Can you work these out from the model? Positions are in its coordinate system, mm. A direction names the side the tool comes from. Give positions to 0.01 mm unless a question says otherwise; leave off trailing zeros. Return JSON: item names as keys, results as strings.
```python
from build123d import *

# Parameters (mm, degrees)
SKETCH1_R           = 1.5
SKETCH1_W           = 8
SKETCH1_H           = 8
BOSS_EXTRUDE1_DEPTH = 8.4


with BuildPart() as part:
    # Sketch1 → Boss-Extrude1 (new body)
    with BuildSketch(Plane(origin=(0, 0, 0), x_dir=(1, 0, 0), z_dir=(0, 1, 0))):
        with BuildLine():
            Line((-160, 31), (-59.260530911, 31))
            ThreePointArc((-59.260530911, 31), (-57, 23.7), (-54.739469089, 31))
            Line((-54.739469089, 31), (77.739469089, 31))
            ThreePointArc((77.739469089, 31), (80, 23.7), (82.260530911, 31))
            Line((82.260530911, 31), (160, 31))
            Line((160, 31), (160, 19.2))
            Line((160, 19.2), (155, 19.2))
            Line((155, 19.2), (155, 20.7))
            Line((155, 20.7), (152, 20.7))
            Line((152, 20.7), (152, 19.2))
            Line((152, 19.2), (150.5, 19.2))
            Line((150.5, 19.2), (150.5, 15.2))
            Line((150.5, 15.2), (152, 15.2))
            Line((152, 15.2), (152, 13.7))
            Line((152, 13.7), (155, 13.7))
            Line((155, 13.7), (155, 15.2))
            Line((155, 15.2), (160, 15.2))
            Line((160, 15.2), (160, 7.248623706))
            Line((160, 7.248623706), (168, 7.248623706))
            Line((168, 7.248623706), (168, -0.751376294))
            Line((168, -0.751376294), (160, -0.751376294))
            Line((160, -0.751376294), (160, -7))
            Line((160, -7), (155, -7))
            Line((155, -7), (155, -5.5))
            Line((155, -5.5), (152, -5.5))
            Line((152, -5.5), (152, -7))
            Line((152, -7), (150.5, -7))
            Line((150.5, -7), (150.5, -11))
            Line((150.5, -11), (152, -11))
            Line((152, -11), (152, -12.5))
            Line((152, -12.5), (155, -12.5))
            Line((155, -12.5), (155, -11))
            Line((155, -11), (160, -11))
            Line((160, -11), (160, -16.2))
            Line((160, -16.2), (168, -16.2))
            Line((168, -16.2), (168, -24.2))
            Line((168, -24.2), (160, -24.2))
            Line((160, -24.2), (160, -31))
            Line((160, -31), (-160, -31))
            Line((-160, -31), (-160, -24.2))
            Line((-160, -24.2), (-168, -24.2))
            Line((-168, -24.2), (-168, -16.2))
            Line((-168, -16.2), (-160, -16.2))
            Line((-160, -16.2), (-160, -11))
            Line((-160, -11), (-155, -11))
            Line((-155, -11), (-155, -12.5))
            Line((-155, -12.5), (-152, -12.5))
            Line((-152, -12.5), (-152, -11))
            Line((-152, -11), (-150.5, -11))
            Line((-150.5, -11), (-150.5, -7))
            Line((-150.5, -7), (-152, -7))
            Line((-152, -7), (-152, -5.5))
            Line((-152, -5.5), (-155, -5.5))
            Line((-155, -5.5), (-155, -7))
            Line((-155, -7), (-160, -7))
            Line((-160, -7), (-160, -0.751376294))
            Line((-160, -0.751376294), (-168, -0.751376294))
            Line((-168, -0.751376294), (-168, 7.248623706))
            Line((-168, 7.248623706), (-160, 7.248623706))
            Line((-160, 7.248623706), (-160, 15.2))
            Line((-160, 15.2), (-155, 15.2))
            Line((-155, 15.2), (-155, 13.7))
            Line((-155, 13.7), (-152, 13.7))
            Line((-152, 13.7), (-152, 15.2))
            Line((-152, 15.2), (-150.5, 15.2))
            Line((-150.5, 15.2), (-150.5, 19.2))
            Line((-150.5, 19.2), (-152, 19.2))
            Line((-152, 19.2), (-152, 20.7))
            Line((-152, 20.7), (-155, 20.7))
            Line((-155, 20.7), (-155, 19.2))
            Line((-155, 19.2), (-160, 19.2))
            Line((-160, 19.2), (-160, 31))
        make_face()
        with Locations((87.1, 27.7)):
            Circle(SKETCH1_R, mode=Mode.SUBTRACT)
        with Locations((72.9, 27.7)):
            Circle(SKETCH1_R, mode=Mode.SUBTRACT)
        with Locations((-49.9, 27.7)):
            Circle(SKETCH1_R, mode=Mode.SUBTRACT)
        with Locations((-64.1, 27.7)):
            Circle(SKETCH1_R, mode=Mode.SUBTRACT)
        with Locations((11.5, 26)):
            Circle(SKETCH1_R, mode=Mode.SUBTRACT)
        with Locations((11.5, -9.4)):
            Circle(SKETCH1_R, mode=Mode.SUBTRACT)
        with Locations((11.5, -0.4)):
            Rectangle(SKETCH1_W, SKETCH1_H, mode=Mode.SUBTRACT)
        with Locations((11.5, 16.2)):
            Rectangle(SKETCH1_W, SKETCH1_H, mode=Mode.SUBTRACT)
    extrude(amount=BOSS_EXTRUDE1_DEPTH)


solid = part.part
```
1. Thinking about a two-plate mould opening in X: for faces 1 (the face through (2, 0, 0)), 2 (the face through (7.5, 4, -16)), 3 (the face through (160, 4, 14)), which applies, +X half, -X half, draft (parallel to the pull), parting line (faces both ways), or undercut?
Checks:
{"face 1": "draft", "face 2": "undercut", "face 3": "+X half"}
2. On a 3-axis mill with a long thin cutter (end or side, diameter ignored), from which of +Z, -Z, +X, -X, +Y, -Y can I reach the whole of each face in a straight line? I mean faces 4 (the face through (160, 4, -11)), 5 (the face through (-164, 4, 0.751)), 6 (the face through (-160, 4, -25)), 7 (the face through (164, 4, 0.751)). Say none if no direction works.
Checks:
{"face 4": "-Z, +X, +Y, -Y", "face 5": "-X, +Y, -Y", "face 6": "-Z, -X, +Y, -Y", "face 7": "+X, +Y, -Y"}
3. Suppose I cut it at A-A (y = 6). State how many separate pieces and enclosed holes the cut face has, plus the area to 3 significant figures.
Checks:
{"separate pieces": "1", "enclosed holes": "8", "area": "19,600 mm^2"}
4. If I drill on L1, parallel to X at y = 6.25, z = 2.5; L2, parallel to X at y = 6.75, z = -15.5; L3, parallel to X at y = 1.75, z = -20, over which ranges is the centre line in solid material (lowest first)? Write a range as [from, to].
Checks:
{"L1": "[-160, 7.5], [15.5, 160]", "L2": "[-150.5, 7.5], [15.5, 150.5]", "L3": "[-160, -155], [-152, 7.5], [15.5, 152], [155, 160]"}
5. For pin 1 Ø3.5 at (y, z) = (3.5, 29) entering from -X; pin 2 Ø1.6 at (y, z) = (6, -14.5) entering from +X, each with a flat end and sliding along its axis, tell me the tip position at first contact or that it passes through.
Checks:
{"pin 1": "x = -160", "pin 2": "x = 160"}
